Here's the drawing with two shaded views (mm, measured from the low corner). I have some questions. Round coordinates to 2 decimals unless told otherwise and drop trailing zeros. Order: outer loops, then holes, each group sorted by start corner. A loop starts at its lowest first (then second) coordinate and runs counter-clockwise, first axis right, second up.
Q1. If we section it at C-C (z = 166): Please give me the cut outline in (x, y).
Q2. If we section it at D-D (x = 42): Please give me the cut outline in (y, z).
Q3. If we section it at A-A (z = 212): Please give me the cut outline in (x, y).
Q4. Will these pins go through, and if not, where does the flat tip stop? P1, Ø1, axis at x = 38, y = 15.5, coming from the -Z side; P2, Ø7, axis at x = 24.5, z = 214, coming from the +Y side; P3, Ø5, axis at x = 23, z = 212, coming from the +Y side.
Q5. If I drill on line 1 (Z direction, x = 34.5, y = 4.25); line 2 (Z direction, x = 23, y = 6.5); line 3 (X direction, y = 1.5, z = 174.5), over which ranges is the centre line in solid material (lowest first)?
Q6. If we section it at B-B (x = 23): Please give me the cut outline in (y, z).
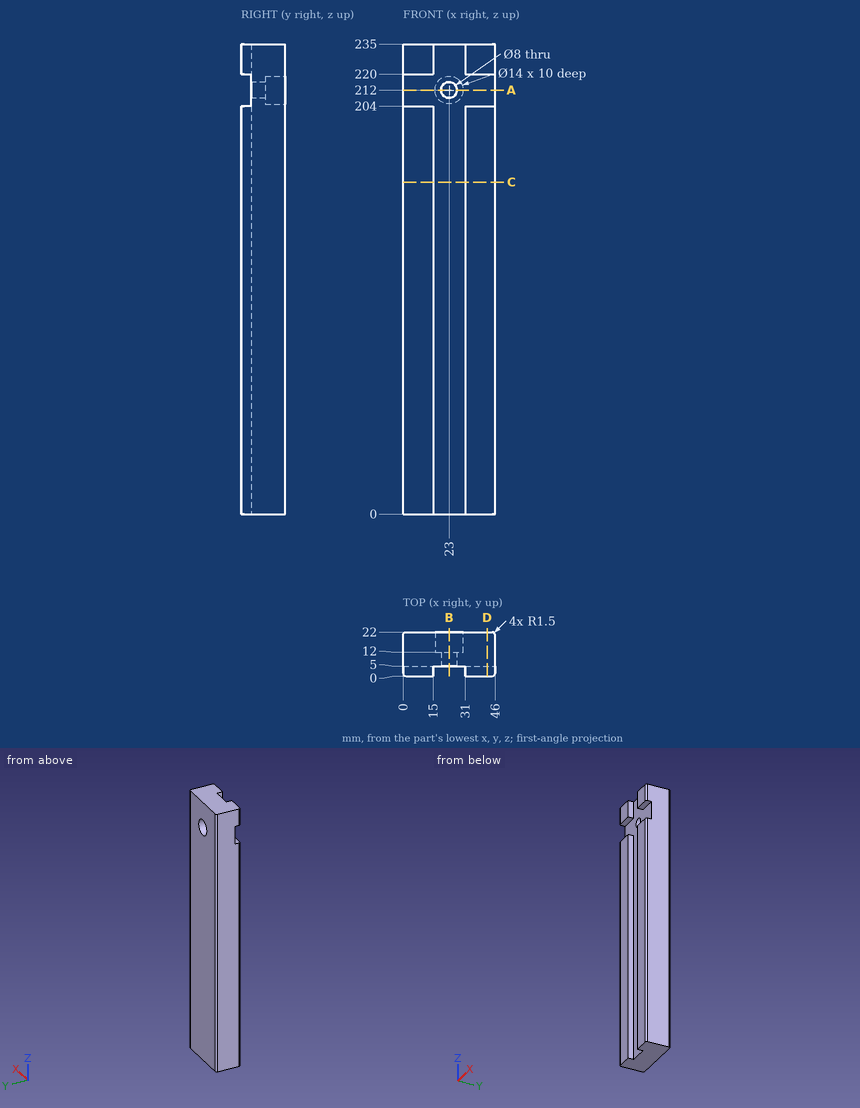
Solution:
1. outline: (0, 1.5) arc R1.5 ccw to (1.5, 0) - (15, 0) - (15, 5) - (31, 5) - (31, 0) - (44.5, 0) arc R1.5 ccw to (46, 1.5) - (46, 20.5) arc R1.5 ccw to (44.5, 22) - (1.5, 22) arc R1.5 ccw to (0, 20.5) - close
2. outline: (0, 0) - (22, 0) - (22, 235) - (0, 235) - (0, 220) - (5, 220) - (5, 204) - (0, 204) - close
3. outline: (0, 5) - (19, 5) - (19, 12) - (16, 12) - (16, 22) - (1.5, 22) arc R1.5 ccw to (0, 20.5) - close; (27, 5) - (46, 5) - (46, 20.5) arc R1.5 ccw to (44.5, 22) - (30, 22) - (30, 12) - (27, 12) - close
4. P1: stops at z = 0
4. P2: stops at y = 12
4. P3: passes through
5. line 1: z = 0 to 204, 220 to 235
5. line 2: z = 0 to 208, 216 to 235
5. line 3: x = 0 to 15, 31 to 46
6. outline: (5, 0) - (22, 0) - (22, 205) - (12, 205) - (12, 208) - (5, 208) - close; (5, 216) - (12, 216) - (12, 219) - (22, 219) - (22, 235) - (5, 235) - close
